```python
from build123d import *

# Parameters (mm, degrees)
SKETCH003_R     = 70
PAD001_DEPTH    = 26
SKETCH004_R     = 42.5
PAD002_DEPTH    = 315
SKETCH005_R     = 35
POCKET002_DEPTH = 315


with BuildPart() as part:
    # Sketch003 → Pad001 (new body)
    with BuildSketch(Plane.XY):
        Circle(SKETCH003_R)
    extrude(amount=PAD001_DEPTH)

    # Sketch004 (on Face3 of Pad001) → Pad002 (join)
    with BuildSketch(Plane.XY.offset(26)):
        Circle(SKETCH004_R)
    extrude(amount=PAD002_DEPTH)

    # Sketch005 (on Face5 of Pad002) → Pocket002 (cut)
    with BuildSketch(Plane.XY.offset(341)):
        Circle(SKETCH005_R)
    extrude(amount=-POCKET002_DEPTH, mode=Mode.SUBTRACT)


with BuildPart() as part_1:
    # Body001 placement: moved
    add(part.part.moved(Location((0, 445, 45))))


solid = part_1.part
```
Input: part model. Units: mm. Frame: model coordinates. A direction names the side the tool comes from. Round coordinates to 2 decimals unless told otherwise and drop trailing zeros. Loops run counter-clockwise (first coordinate to the right, second up) from the corner with the lowest first, then second, coordinate; pieces in that order, holes last. Notation, with made-up numbers: M 18,-9 L 39,-9 A29 cw 39,15 Z; hole C 8.25,41 d1. An arc over 180 degrees is marked long. Answer in a Markdown table with one row per item. Add a question column.
1. Section B-B (x = 0). Output: boundary loops of the cut face in (y, z).
2. Section D-D (x = -51). Output: boundary loops of the cut face in (y, z).
3. Ray query, probe 1 along Y at (x, z) = (0, 150.5); probe 2 along Z at (x, y) = (-51.5, 408.5); probe 3 along Y at (x, z) = (16, 196). Return the intervals inside material, ascending.
4. Section C-C (z = 78). Output: boundary loops of the cut face in (x, y).
5. Set-up query: faces 1 (the face through (-5.53, 487.14, 226.3)), 2 (the face through (6, 480, 386)). Return all of +Z, -Z, +X, -X, +Y, -Y with unobstructed straight access to the full face (end or side cutting, diameter ignored); none if empty.
6. Contact query for flat-ended pins moving along their axis: pin 1 (5 mm diameter, centred on y = 481, z = 147, fed in from +X); pin 2 (4 mm diameter, centred on y = 474.5, z = 156.5, fed in from -X); pin 3 (5 mm diameter, centred on x = -9.5, z = 141, fed in from +Y). Output: stop coordinate, or through.
7. Section A-A (y = 445). Output: boundary loops of the cut face in (x, z), and give its area (4 significant figures).
8. Mould query, pull axis X, two halves, no side actions, for faces 3 (the face through (-9.113, 514.404, 57.818)), 4 (the face through (-4.56, 479.7, 230.7)), 5 (the face through (46, 446, 71)). Classes: released by +X, released by -X, zero draft, split by the parting line, or undercut.
Values follow:
| question | item | result |
|---|---|---|
| 1 | outline | M 375,45 L 515,45 L 515,71 L 487.5,71 L 487.5,386 L 480,386 L 480,71 L 410,71 L 410,386 L 402.5,386 L 402.5,71 L 375,71 Z |
| 2 | outline | M 397.05,45 L 492.95,45 L 492.95,71 L 397.05,71 Z |
| 3 | probe 1 | 402.5 to 410, 480 to 487.5 |
| 3 | probe 2 | 45 to 71 |
| 3 | probe 3 | 405.63 to 413.87, 476.13 to 484.37 |
| 4 | outline | C 0,445 d85; hole C 0,445 d70 |
| 5 | face 1 | +Z |
| 5 | face 2 | +Z, +X, -X, +Y, -Y |
| 6 | pin 1 | x = 26.15 |
| 6 | pin 2 | x = -32.4 |
| 6 | pin 3 | y = 486.92 |
| 7 | outline | M -70,45 L 70,45 L 70,71 L 42.5,71 L 42.5,386 L 35,386 L 35,71 L -35,71 L -35,386 L -42.5,386 L -42.5,71 L -70,71 Z |
| 7 | area | 8,365 mm^2 |
| 8 | face 3 | split by the parting line |
| 8 | face 4 | undercut |
| 8 | face 5 | zero draft |
